Part model, mm, in its own coordinate system. A direction names the side the tool comes from. Coordinates: 2 decimals unless noted, no trailing zeros. Order: outer loops, then holes, each group sorted by start corner. A loop starts at its lowest first (then second) coordinate and runs counter-clockwise, first axis right, second up.
from build123d import *

# Parameters (mm, degrees)
F0_R     = 29.21
F1_DEPTH = 25.908
F2_R     = 39.37
F3_DEPTH = 38.1
F4_T     = -5.08
F5_SIZE  = 8.128
F7_D     = 6.35
F7_DEPTH = 38.101


with BuildPart() as f1:
    # F0 (on Top) → F1 (new body)
    with BuildSketch(Plane.XY):
        Circle(F0_R)
    extrude(amount=-F1_DEPTH)

    # F2 (on Top) → F3 (join)
    with BuildSketch(Plane.XY):
        Circle(F2_R)
    extrude(amount=F3_DEPTH)

    # F4
    f4_openings = [f1.faces().sort_by_distance(p)[0] for p in [
        (0, 0, 38.1),
        (0, 0, -25.908),
    ]]
    offset(amount=F4_T, openings=f4_openings, kind=Kind.INTERSECTION)

    # F5
    f5_edges = [f1.edges().sort_by_distance(p)[0] for p in [
        (-39.37, 0, 0),
    ]]
    chamfer(f5_edges, length=F5_SIZE)

    # F7 (through all, one way)
    with BuildSketch(Plane(origin=(0, 0, 0), x_dir=(1, 0, 0), z_dir=(0, 0, -1))):
        with Locations((25.4209353007, 18.1614595349)):
            Circle(F7_D / 2)
    extrude(amount=-F7_DEPTH, mode=Mode.SUBTRACT)


solid = f1.part
Q1. Cut at A-A on x = 0. Write the cut outline in (y, z), and give its area (3 significant figures).
Results list:
outline: (-39.37, 8.13) - (-31.24, 0) - (-29.21, 0) - (-29.21, -25.91) - (-24.13, -25.91) - (-24.13, 5.08) - (-34.29, 5.08) - (-34.29, 38.1) - (-39.37, 38.1) - close; (24.13, -25.91) - (29.21, -25.91) - (29.21, 0) - (31.24, 0) - (39.37, 8.13) - (39.37, 38.1) - (34.29, 38.1) - (34.29, 5.08) - (24.13, 5.08) - close
area: 687 mm2
Q2. Wall check: line 1 along Z through (x, y) = (-30.5, -2); line 2 along X through (y, z) = (-1, 33.5); line 3 along Y through (x, z) = (-23.5, 5.5). Give the ranges that are in metal, low to high.
Results list:
line 1: z = 0 to 5.08
line 2: x = -39.36 to -34.28, 34.28 to 39.36
line 3: y = -28.24 to -24.97, 24.97 to 28.24
Q3. Cut at B-B on z = -19.5. Write the cut outline in (x, y), and give its area (3 significant figures).
Results list:
outline: circle Ø58.42 at (0, 0); hole circle Ø48.26 at (0, 0)
area: 851 mm2
Q4. Pin check, flat tips, straight feed: pin 1 Ø6 at (y, z) = (20.5, -1) entering from +X; pin 2 Ø0.8 at (x, y) = (24, -16.5) entering from +Z; pin 3 Ø6 at (x, z) = (0.5, -16.5) entering from +Y; pin 4 Ø20.5 at (x, y) = (-11, -4.5) entering from +Z. Stop position of each tip, or through.
Results list:
pin 1: stops at x = 26.79
pin 2: stops at z = 0
pin 3: stops at y = 29.21
pin 4: passes through
Q5. Mould opens along Y. For faces 4 (the face through (-23.318, 21.382, 0.395)), 5 (the face through (-28, 9, 0)), 6 (the face through (23, -17, 0)) say: pulls with the +Y half, pulls with the -Y half, needs draft (parallel to the pull), parting line crosses it, or undercut.
Results list:
face 4: parting line crosses it
face 5: needs draft
face 6: undercut
Q6. Which spindle directions (+Z, -Z, +X, -X, +Y, -Y) get a long thin tool onto all of the face, cutting with end or side? Do faces 1 (the face through (12.97, 20.35, -10.2)), 2 (the face through (-21.53, 19.74, -12.77)), 3 (the face through (27.63, -20.44, 10.49)). Say none if no direction does.
Results list:
face 1: +Z, -Z
face 2: -Z
face 3: +Z
